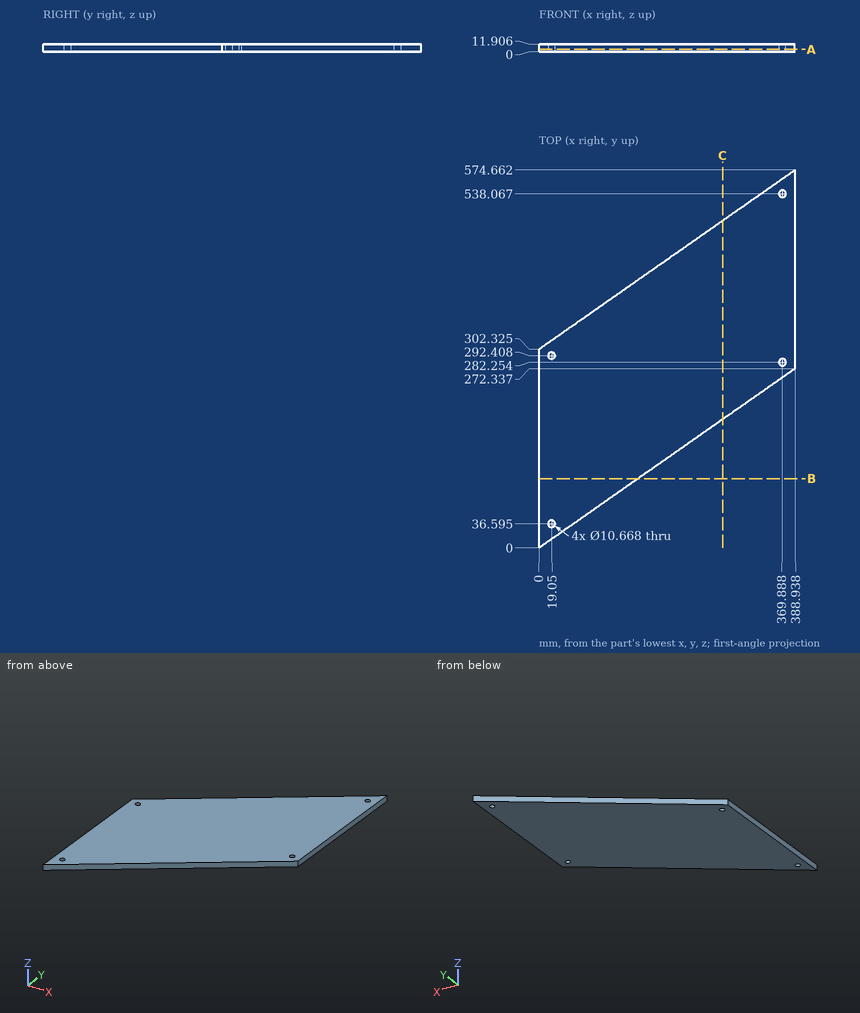
Verification items for this drawing (mm, ordinates from the low corner). Give positions to 0.01 mm unless a question says otherwise; leave off trailing zeros. Loops run counter-clockwise (first coordinate to the right, second up) from the corner with the lowest first, then second, coordinate; pieces in that order, holes last. Notation, with made-up numbers: M 80,-20.5 L 95,-20.5 A16 cw 95,-14.5 Z; hole C 88,36.5 d10. An arc over 180 degrees is marked long. Write item = value, one per line. Start each with the question number.
1. Go/stop test with flat-tipped pins: P1, Ø8.5, axis at x = 369.89, y = 282.25, coming from the +Z side; P2, Ø5, axis at x = 159.5, z = 8, coming from the -Y side. Record where each tip stops, or that it passes through.
2. Thickness scan on probe 1 along Y at (x, z) = (19.05, 2.75) (1 decimal); probe 2 along X at (y, z) = (493.5, 5.5) (1 decimal); probe 3 along X at (y, z) = (329.5, 3) (1 decimal). Record the ranges inside material, lowest first.
3. Section check C-C, the plane x = 279. Enter the section's corners in (y, z).
4. Section check B-B, the plane y = 105.5. Enter the section's corners in (x, z), plus the area to 3 significant figures.
5. Section check A-A, the plane z = 3.75. Give the number of separate pieces and of enclosed holes in the cut face, plus the area to 3 significant figures.
Values follow:
q1.P1 = through
q1.P2 = 109.93
q2.probe_1 = 13.3 to 31.3, 41.9 to 287.1, 297.7 to 315.7
q2.probe_2 = 273 to 388.9
q2.probe_3 = 38.8 to 388.9
q3.outline = M 195.36,0 L 497.68,0 L 497.68,11.91 L 195.36,11.91 Z
q4.outline = M 0,0 L 150.67,0 L 150.67,11.91 L 0,11.91 Z
q4.area = 1,790 mm^2
q5.separate_pieces = 1
q5.enclosed_holes = 4
q5.area = 117,000 mm^2
